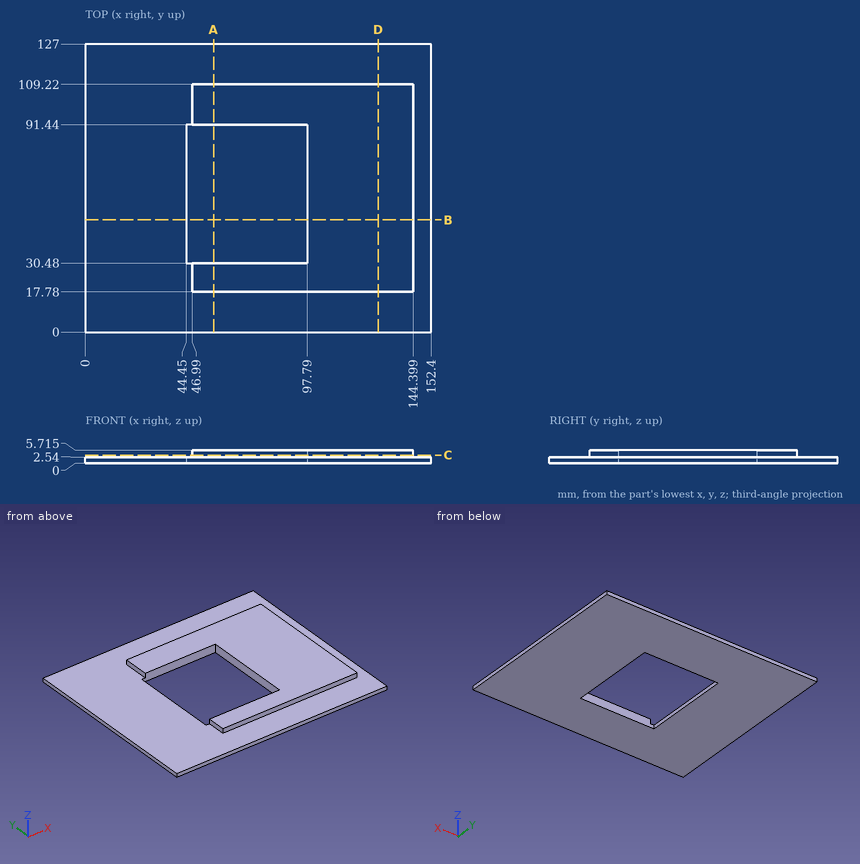
Design review of the part shown in the three views and the two pictorial views. Dimensions are in mm from the part's minimum x, y and z. Give positions to 0.01 mm unless a question says otherwise; leave off trailing zeros. Loops run counter-clockwise (first coordinate to the right, second up) from the corner with the lowest first, then second, coordinate; pieces in that order, holes last. Notation, with made-up numbers: (52, 12) -> (56, 12) arc R26 ccw to (56, 40) -> close; hole circle Ø4 at (15, 18). An arc over 180 degrees is marked (long way). Write each question's results on one line, items separated by ' | '.
Q1. Take a section at B-B, the plane y = 49.5. Write out the cut boundary in (x, z) (3 decimals).
Reply:
outline: (0, 0) -> (44.45, 0) -> (44.45, 2.54) -> (0, 2.54) -> close; (97.79, 0) -> (152.4, 0) -> (152.4, 2.54) -> (144.399, 2.54) -> (144.399, 5.715) -> (97.79, 5.715) -> close
Q2. Take a section at D-D, the plane x = 129. Write out the cut boundary in (y, z) (3 decimals).
Reply:
outline: (0, 0) -> (127, 0) -> (127, 2.54) -> (109.22, 2.54) -> (109.22, 5.715) -> (17.78, 5.715) -> (17.78, 2.54) -> (0, 2.54) -> close
Q3. Take a section at A-A, the plane x = 56.5. Write out the cut boundary in (y, z) (3 decimals).
Reply:
outline: (0, 0) -> (30.48, 0) -> (30.48, 5.715) -> (17.78, 5.715) -> (17.78, 2.54) -> (0, 2.54) -> close; (91.44, 0) -> (127, 0) -> (127, 2.54) -> (109.22, 2.54) -> (109.22, 5.715) -> (91.44, 5.715) -> close
Q4. Take a section at C-C, the plane z = 3.5. Write out the cut boundary in (x, y), plus the area to 3 significant figures.
Reply:
outline: (46.99, 17.78) -> (144.4, 17.78) -> (144.4, 109.22) -> (46.99, 109.22) -> (46.99, 91.44) -> (97.79, 91.44) -> (97.79, 30.48) -> (46.99, 30.48) -> close | area: 5,810 mm²
Q5. Wall thickness on L1, parallel to X at y = 81.5, z = 0.6; L2, parallel to Y at x = 92.5, z = 1.95; L3, parallel to Y at x = 84, z = 3.4: over which ranges is each line inside the solid? List them lowest first.
Reply:
L1: x = 0 to 44.45, 97.79 to 152.4 | L2: y = 0 to 30.48, 91.44 to 127 | L3: y = 17.78 to 30.48, 91.44 to 109.22
Q6. For pin 1 Ø2.5 at (x, z) = (76, 4) entering from +Y; pin 2 Ø1.6 at (y, z) = (97.5, 4.5) entering from -X; pin 3 Ø1 at (y, z) = (56.5, 4) entering from +X, all flat-tipped, find the tip position at first contact; note any pin that passes through.
Reply:
pin 1: stops at y = 109.22 | pin 2: stops at x = 46.99 | pin 3: stops at x = 144.4
